Autodesk Fusion 360 part; units mm, degrees
sketch "Sketch1" plane through (0, 0, 0) normal (0, 0, 1) x (1, 0, 0)
  circle A0 centre (0, 0) radius 72.5
  line L0 (0, 0) -> (-170.1079, 0) construction
  arc A1 (-7.5, 57.0088) -> (-57.0088, 7.5) centre (0, 0) ccw
  line L1 (0, 0) -> (0, 73.0172) construction
  line L2 (-57.0088, 7.5) -> (-18.5405, 7.5)
  line L3 (-7.5, 57.0088) -> (-7.5, 18.5405)
  circle A2 centre (0, 0) radius 5
  arc A3 (-7.5, 18.5405) -> (-18.5405, 7.5) centre (0, 0) ccw
  dimension "d2" = 145
  dimension "d9" = 90
  dimension "d10" = 7.5
  dimension "d11" = 7.5
  dimension "d12" = 15
  dimension "d13" = 10
  dimension "d15" = 15
extrude "Extrude1" add sketch "Sketch1" along normal blind 20 contours A0 | A1 L2 L3 A3 | A2
extrude "Extrude2" cut sketch "Sketch1" along normal up to surface (20 mm away) contours A1 L2 L3 A3
extrude "Extrude3" cut sketch "Sketch1" along normal up to surface (20 mm away) draft 1 contours A2
pattern_circular "C-Pattern1" count 4 over 360 about axis through (0, 0, 1.75) along (0, 0, 1) of "Extrude2"
equation "d2 = OverallDiameter"
equation "HubHoleDiameter = 10 mm"
equation "HubWallThickness = 15 mm"
equation "OverallDiameter = 145 mm"
equation "PartHeight = 20 mm"
equation "d9 = ( 360 / NumberOfSPokes ) * 1 deg"
equation "d10 = HubWallThickness / 2"
equation "d11 = HubWallThickness / 2"
equation "d12 = HubWallThickness"
equation "d13 = HubHoleDiameter"
equation "d15 = HubWallThickness"
equation "d16 = PartHeight"
equation "HubHoleTaperAngle = 1 deg"
equation "d22 = HubHoleTaperAngle"
The model under review builds one solid part; all positions refer to its coordinate system, in mm. A direction names the side the tool comes from. Round coordinates to 2 decimals unless told otherwise and drop trailing zeros. Order: outer loops, then holes, each group sorted by start corner. A loop starts at its lowest first (then second) coordinate and runs counter-clockwise, first axis right, second up. Notation, with made-up numbers: (19, 9) -> (68, 9) arc R17 ccw to (68, 17) -> close; hole circle Ø5 at (-35.75, 44.25). An arc over 180 degrees is marked (long way). Write item = value, one per line. Start each with the question number.
Item 1: Consider section A-A on x = -44. Write out the cut boundary in (y, z), plus the area to 3 significant figures.
Item 2: Clearance check with flat-ended pins moving along their axes: pin 1 Ø12 at (y, z) = (-24, 9) entering from +X; pin 2 Ø6 at (x, z) = (31.5, 6.5) entering from -Y; pin 3 Ø3 at (x, z) = (56.5, 11.5) entering from -Y. State where each tip first meets the part, or that it passes through.
Item 3: For faces 4 (the face through (15, 1, 0)), 5 (the face through (-4.11, -3.15, 10.14)), 6 (the face through (-14.063, -14.221, 9.86)), list the 3-axis set-ups (+Z, -Z, +X, -X, +Y, -Y) from which the entire face can be reached by the end or side of a thin tool; tool diameter is ignored.
Item 4: For line 1 along X through (y, z) = (24, 13); line 2 along X through (y, z) = (-49, 11); line 3 along Y through (x, z) = (17.5, 9.25), list the stretches that pass through material, from the lowest coordinate up.
Item 5: Consider section B-B on z = 16. Write out the cut boundary in (x, y), plus the area to 3 significant figures.
Item 6: Consider section C-C on x = -29. Write out the cut boundary in (y, z).
Item 7: Consider section D-D on z = 6.75. Write out the cut boundary in (x, y).
Item 8: Mouldability with a two-part tool opening along Y and no side actions: class faces 1 (the face through (-38, -7.5, 10)), 2 (the face through (15, 1, 20)), 3 (the face through (69.15, -21.78, 9.86)) as released by +Y, released by -Y, zero draft, split by the parting line, or undercut.
Conclusion:
q1.outline = (-57.62, 0) -> (-37.02, 0) -> (-37.02, 20) -> (-57.62, 20) -> close; (-7.5, 0) -> (7.5, 0) -> (7.5, 20) -> (-7.5, 20) -> close; (37.02, 0) -> (57.62, 0) -> (57.62, 20) -> (37.02, 20) -> close
q1.area = 1,120 mm2
q2.pin_1 = 70.23
q2.pin_2 = -66.66
q2.pin_3 = -47.24
q3.face_4 = -Z, +X, -X, +Y, -Y
q3.face_5 = +Z
q3.face_6 = +Z, -Z
q4.line_1 = -68.41 to -52.25, -7.5 to 7.5, 52.25 to 68.41
q4.line_2 = -53.43 to -30.09, -7.5 to 7.5, 30.09 to 53.43
q4.line_3 = -70.36 to -54.77, -9.68 to 9.68, 54.77 to 70.36
q5.outline = circle Ø145 at (0, 0); hole (-57.01, -7.5) arc R57.5 ccw to (-7.5, -57.01) -> (-7.5, -18.54) arc R20 cw to (-18.54, -7.5) -> close; hole (-57.01, 7.5) -> (-18.54, 7.5) arc R20 cw to (-7.5, 18.54) -> (-7.5, 57.01) arc R57.5 ccw to start; hole circle Ø10.56 at (0, 0); hole (7.5, -57.01) arc R57.5 ccw to (57.01, -7.5) -> (18.54, -7.5) arc R20 cw to (7.5, -18.54) -> close; hole (7.5, 18.54) arc R20 cw to (18.54, 7.5) -> (57.01, 7.5) arc R57.5 ccw to (7.5, 57.01) -> close
q5.area = 9,560 mm2
q6.outline = (-66.45, 0) -> (-49.65, 0) -> (-49.65, 20) -> (-66.45, 20) -> close; (-7.5, 0) -> (7.5, 0) -> (7.5, 20) -> (-7.5, 20) -> close; (49.65, 0) -> (66.45, 0) -> (66.45, 20) -> (49.65, 20) -> close
q7.outline = circle Ø145 at (0, 0); hole (-57.01, -7.5) arc R57.5 ccw to (-7.5, -57.01) -> (-7.5, -18.54) arc R20 cw to (-18.54, -7.5) -> close; hole (-57.01, 7.5) -> (-18.54, 7.5) arc R20 cw to (-7.5, 18.54) -> (-7.5, 57.01) arc R57.5 ccw to start; hole circle Ø10.24 at (0, 0); hole (7.5, -57.01) arc R57.5 ccw to (57.01, -7.5) -> (18.54, -7.5) arc R20 cw to (7.5, -18.54) -> close; hole (7.5, 18.54) arc R20 cw to (18.54, 7.5) -> (57.01, 7.5) arc R57.5 ccw to (7.5, 57.01) -> close
q8.face_1 = undercut
q8.face_2 = zero draft
q8.face_3 = split by the parting line
